Design review of the part built by this model. Coordinates are the model's own, in mm. A direction names the side the tool comes from. Coordinates: 2 decimals unless noted, no trailing zeros. Loops run counter-clockwise (first coordinate to the right, second up) from the corner with the lowest first, then second, coordinate; pieces in that order, holes last. Notation, with made-up numbers: (77, 29.25) -> (83, 29.25) arc R16 ccw to (83, 53.25) -> close; hole circle Ø9 at (9.5, 79.5). An arc over 180 degrees is marked (long way). Answer in a Markdown table with one row per item.
```python
from build123d import *

# Parameters (mm, degrees)
SKETCH1_R           = 2.1
SKETCH1_R_2         = 1.75
SKETCH1_R_3         = 1.35
BOSS_EXTRUDE1_DEPTH = 5


with BuildPart() as part:
    # Sketch1 → Boss-Extrude1 (new body)
    with BuildSketch(Plane.XY):
        with BuildLine():
            Line((-62.05384494, 14.663645746), (-65.886192563, -7.070677654))
            ThreePointArc((-65.886192563, -7.070677654), (-64.967386661, -10.499707961), (-61.75, -12))
            Line((-61.75, -12), (40.25, -12))
            Line((40.25, -12), (40.25, 50.37))
            ThreePointArc((40.25, 50.37), (37.429438303, 57.179438303), (30.62, 60))
            Line((30.62, 60), (-52.12, 60))
            ThreePointArc((-52.12, 60), (-58.929438303, 57.179438303), (-61.75, 50.37))
            Line((-61.75, 50.37), (-61.75, 18.1366093))
            ThreePointArc((-61.75, 18.1366093), (-61.826106038, 16.393494445), (-62.05384494, 14.663645746))
        make_face()
        Circle(SKETCH1_R, mode=Mode.SUBTRACT)
        with Locations((-48.75, 50.37)):
            Circle(SKETCH1_R_2, mode=Mode.SUBTRACT)
        with Locations((32.75, -7.8)):
            Circle(SKETCH1_R_3, mode=Mode.SUBTRACT)
        with Locations((2.25, 50.37)):
            Circle(SKETCH1_R_2, mode=Mode.SUBTRACT)
        with Locations((-61.75, -7.8)):
            Circle(SKETCH1_R_3, mode=Mode.SUBTRACT)
        with Locations((-4.75, -7.8)):
            Circle(SKETCH1_R_3, mode=Mode.SUBTRACT)
        with Locations((0, 20)):
            Circle(SKETCH1_R, mode=Mode.SUBTRACT)
        with BuildLine():
            Line((-47.5, -4.5), (-42.5, -4.5))
            ThreePointArc((-42.5, -4.5), (-40.5, -6.5), (-42.5, -8.5))
            Line((-42.5, -8.5), (-47.5, -8.5))
            ThreePointArc((-47.5, -8.5), (-49.5, -6.5), (-47.5, -4.5))
        make_face(mode=Mode.SUBTRACT)
    extrude(amount=BOSS_EXTRUDE1_DEPTH)


solid = part.part
```
(1) Tool access review of faces 4 (the cylindrical face through (-49.5, -6.5, 2.5)), 5 (the flat face through (-14, 25, 5)): name each direction out of +Z, -Z, +X, -X, +Y, -Y from which nothing blocks a thin tool from reaching the whole face with its end or side.
Evaluation:
| item | result |
|---|---|
| face 4 | +Z, -Z |
| face 5 | +Z, +X, -X, +Y, -Y |
(2) Draft analysis for pull direction Y (two halves, no side actions). For faces 1 (the cylindrical face through (37.504, 57.104, 2.465)), 2 (the cylindrical face through (2.022, 52.105, 2.465)), 3 (the flat face through (-61.75, 34, 2)), state which applies: pulls with the +Y half, pulls with the -Y half, needs draft (parallel to the pull), parting line crosses it, or undercut.
Evaluation:
| item | result |
|---|---|
| face 1 | pulls with the +Y half |
| face 2 | undercut |
| face 3 | needs draft |
(3) To check wall thickness, follow probe 1 along X at (y, z) = (46, 4.2); probe 2 along Y at (x, z) = (-48.75, 3.7); probe 3 along Y at (x, z) = (-41, 4.3). State the ranges of each line that lie inside material, in increasing order.
Evaluation:
| item | result |
|---|---|
| probe 1 | x = -61.75 to 40.25 |
| probe 2 | y = -12 to -8.06, -4.94 to 48.62, 52.12 to 60 |
| probe 3 | y = -12 to -7.82, -5.18 to 60 |
(4) For pin 1 (3 mm diameter, centred on x = -4.75, y = -7.8, fed in from +Z); pin 2 (1 mm diameter, centred on y = 29, z = 4.5, fed in from -X), all flat-tipped, find the tip position at first contact; note any pin that passes through.
Evaluation:
| item | result |
|---|---|
| pin 1 | stops at z = 5 |
| pin 2 | stops at x = -61.75 |
(5) Take a section at D-D on y = 34.5. Give the boundary of the cut face in (x, z), and give its area (3 significant figures).
Evaluation:
| item | result |
|---|---|
| outline | (-61.75, 0) -> (40.25, 0) -> (40.25, 5) -> (-61.75, 5) -> close |
| area | 510 mm² |
(6) Take a section at A-A on y = 20. Give the boundary of the cut face in (x, z).
Evaluation:
| item | result |
|---|---|
| outline | (-61.75, 0) -> (-2.1, 0) -> (-2.1, 5) -> (-61.75, 5) -> close; (2.1, 0) -> (40.25, 0) -> (40.25, 5) -> (2.1, 5) -> close |
(7) Take a section at B-B on x = -4.75. Give the boundary of the cut face in (y, z).
Evaluation:
| item | result |
|---|---|
| outline | (-12, 0) -> (-9.15, 0) -> (-9.15, 5) -> (-12, 5) -> close; (-6.45, 0) -> (60, 0) -> (60, 5) -> (-6.45, 5) -> close |
(8) Take a section at C-C on z = 1.5. Count the separate pieces of the cut face and the enclosed holes in it, and give its area (3 significant figures).
Evaluation:
| item | result |
|---|---|
| separate pieces | 1 |
| enclosed holes | 8 |
| area | 7,270 mm² |
